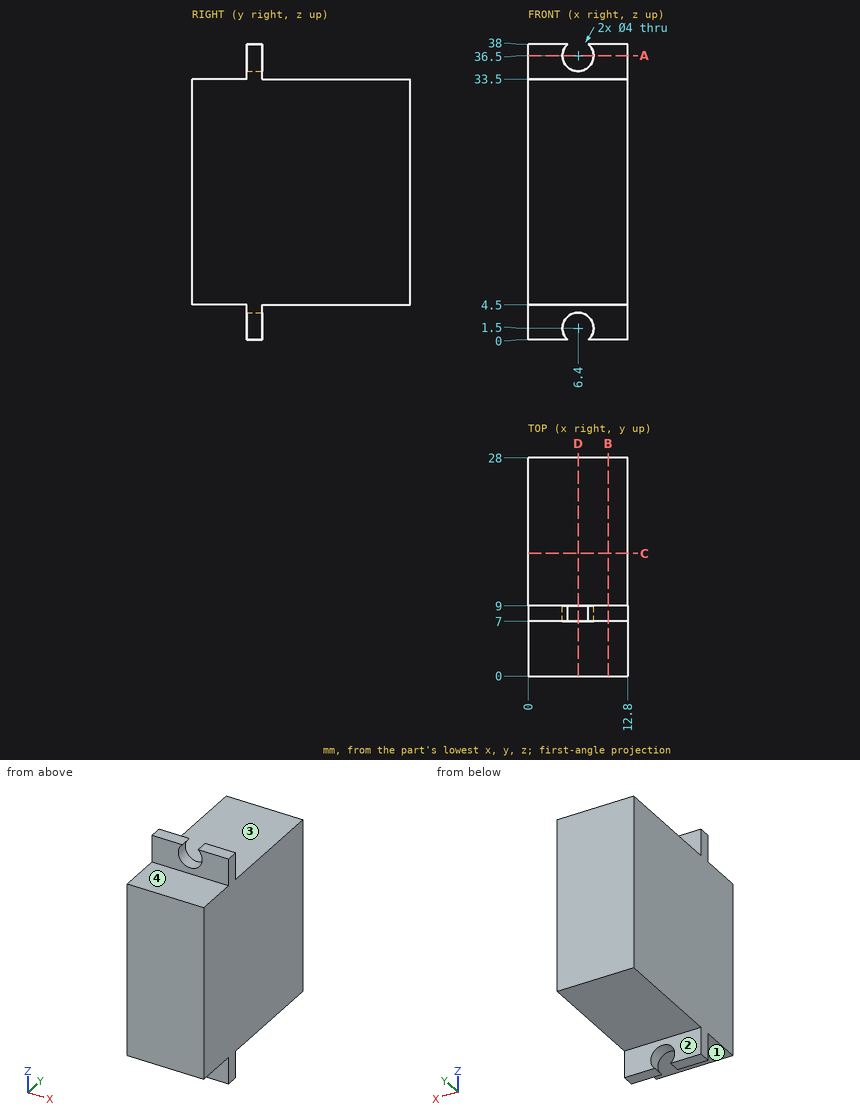
Could you check a few things on this drawing? It's one solid part, dimensions in mm from its lowest x, y, z. A direction names the side the tool comes from. Round coordinates to 2 decimals unless told otherwise and drop trailing zeros. Order: outer loops, then holes, each group sorted by start corner. A loop starts at its lowest first (then second) coordinate and runs counter-clockwise, first axis right, second up. Notation, with made-up numbers: M -2.75,-7.75 L 31.25,-7.75 A14 cw 31.25,17.25 Z; hole C 40.5,-6.75 d1. An arc over 180 degrees is marked long. Return JSON: item names as keys, results as strings. Group by question number.
1. Please list where these lines run through material, in increasing order: probe 1 along X at (y, z) = (7.5, 36.5); probe 2 along Z at (x, y) = (7.5, 20.25); probe 3 along Y at (x, z) = (0.5, 35).
2. If we section it at A-A on z = 36.5: List the corners of the cut face in (x, y) for me, then the cut area to 3 significant figures.
3. I'm going to push flat-ended pins straight in: pin 1 Ø2 at (x, y) = (4, 4.5) entering from -Z; pin 2 Ø4 at (y, z) = (17.5, 10.5) entering from -X; pin 3 Ø3 at (x, y) = (10.5, 13.5) entering from +Z; pin 4 Ø3.5 at (x, z) = (6.5, 37) entering from +Y. Where does each tip first touch, or does it pass through?
4. On a 3-axis mill with a long thin cutter (end or side, diameter ignored), from which of +Z, -Z, +X, -X, +Y, -Y can I reach the whole of each face in a straight line? I mean the marked faces 1, 2, 3 and 4. Say none if no direction works.
5. If we section it at D-D on x = 6.4: List the corners of the cut face in (y, z) for me, then the cut area to 3 significant figures.
6. If we section it at B-B on x = 10.25: List the corners of the cut face in (y, z) for me.
7. If we section it at C-C on y = 15.75: List the corners of the cut face in (x, z) for me, then the cut area to 3 significant figures.
Reply:
{
 "1": {"probe 1": "0 to 4.4, 8.4 to 12.8", "probe 2": "4.5 to 33.5", "probe 3": "7 to 9"},
 "2": {"outline": "M 0,7 L 4.4,7 L 4.4,9 L 0,9 Z; M 8.4,7 L 12.8,7 L 12.8,9 L 8.4,9 Z", "area": "17.6 mm^2"},
 "3": {"pin 1": "z = 4.5", "pin 2": "x = 0", "pin 3": "z = 33.5", "pin 4": "y = 9"},
 "4": {"face 1": "-Z, +X, -X, -Y", "face 2": "-Z, +X, -X, +Y", "face 3": "+Z, +X, -X, +Y", "face 4": "+Z, +X, -X, -Y"},
 "5": {"outline": "M 0,4.5 L 7,4.5 L 7,3.5 L 9,3.5 L 9,4.5 L 28,4.5 L 28,33.5 L 9,33.5 L 9,34.5 L 7,34.5 L 7,33.5 L 0,33.5 Z", "area": "816 mm^2"},
 "6": {"outline": "M 0,4.5 L 7,4.5 L 7,0 L 9,0 L 9,4.5 L 28,4.5 L 28,33.5 L 9,33.5 L 9,38 L 7,38 L 7,33.5 L 0,33.5 Z"},
 "7": {"outline": "M 0,4.5 L 12.8,4.5 L 12.8,33.5 L 0,33.5 Z", "area": "371 mm^2"}
}
